from build123d import *

# Parameters (mm, degrees)
BOSS_EXTRUDE7_DEPTH = 3
SKETCH12_R          = 1.15
CUT_EXTRUDE3_DEPTH  = 75.228296491
SKETCH11_R          = 1.45
CUT_EXTRUDE4_DEPTH  = 75.228296491
SKETCH13_R          = 1.15
CUT_EXTRUDE5_DEPTH  = 75.228296491
FILLET1_R           = 4.7
FILLET2_R           = 3.8


with BuildPart() as part:
    # Sketch10 → Boss-Extrude7 (new body)
    with BuildSketch(Plane.XY):
        Polygon((22.4, 10.2), (62.6, 10.2), (62.6, -10.2), (72, -10.2), (72, 17.8), (8, 17.8), (8, 10.2), (-8, 10.2), (-8, 5), (8, 5), (8, -5), (-8, -5), (-8, -10.2), (22.4, -10.2), align=None)
    extrude(amount=-BOSS_EXTRUDE7_DEPTH)

    # Sketch12 → Cut-Extrude3 (cut, through all)
    with BuildSketch(Plane(origin=(0, 0, 0), x_dir=(-1, 0, 0), z_dir=(0, 0, -1))):
        with Locations((-57.5, 12.7)):
            Circle(SKETCH12_R)
        with Locations((-47.5, 12.7)):
            Circle(SKETCH12_R)
    extrude(amount=CUT_EXTRUDE3_DEPTH, mode=Mode.SUBTRACT)

    # Sketch11 → Cut-Extrude4 (cut, through all)
    with BuildSketch(Plane(origin=(0, 0, 0), x_dir=(-1, 0, 0), z_dir=(0, 0, -1))):
        with Locations((-67.3, -5)):
            Circle(SKETCH11_R)
        with Locations((-17.7, -5)):
            Circle(SKETCH11_R)
        with Locations((-17.7, 5)):
            Circle(SKETCH11_R)
        with Locations((-67.3, 5)):
            Circle(SKETCH11_R)
    extrude(amount=CUT_EXTRUDE4_DEPTH, mode=Mode.SUBTRACT)

    # Sketch13 → Cut-Extrude5 (cut, through all)
    with BuildSketch(Plane.XY):
        with Locations((5, 7.6)):
            Circle(SKETCH13_R)
        with Locations((5, -7.6)):
            Circle(SKETCH13_R)
    extrude(amount=-CUT_EXTRUDE5_DEPTH, mode=Mode.SUBTRACT)

    # Fillet1
    fillet1_edges = [part.edges().sort_by_distance(p)[0] for p in [
        (72, 17.8, -1.5),
        (72, -10.2, -1.5),
    ]]
    fillet(fillet1_edges, radius=FILLET1_R)

    # Fillet2
    fillet2_edges = [part.edges().sort_by_distance(p)[0] for p in [
        (22.4, -10.2, -1.5),
        (-8, -10.2, -1.5),
        (8, 17.8, -1.5),
        (8, 10.2, -1.5),
        (-8, 10.2, -1.5),
    ]]
    fillet(fillet2_edges, radius=FILLET2_R - 0.0001)  # a hair under: the kernel refuses the full size


solid = part.part
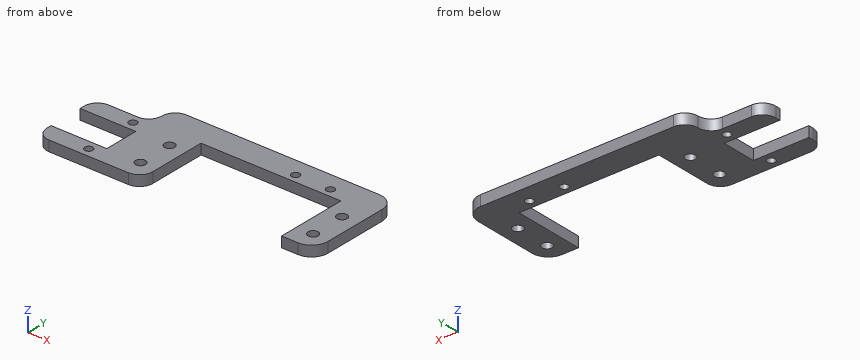
Geometry check sheet. Reference: the model listing, model coordinates, mm. Round coordinates to 2 decimals unless told otherwise and drop trailing zeros. Order: outer loops, then holes, each group sorted by start corner. A loop starts at its lowest first (then second) coordinate and runs counter-clockwise, first axis right, second up. Notation, with made-up numbers: M 76.25,65 L 101.25,65 A15 ccw 101.25,82 Z; hole C 47.25,44.5 d4. An arc over 180 degrees is marked long. Answer in a Markdown table with one row per item. Add a question column.
Item 1: Sectioned sample at D-D, the plane y = 7.6. Enter the section's corners in (x, z).
Item 2: Sectioned sample at C-C, the plane y = -2. Enter the section's corners in (x, z), plus the area to 3 significant figures.
Item 3: Sectioned sample at A-A, the plane x = 57.5. Enter the section's corners in (y, z), plus the area to 3 significant figures.
Item 4: Sectioned sample at B-B, the plane z = -1.5. State how many separate pieces and enclosed holes the cut face has, plus the area to 3 significant figures.
Item 5: Material ranges on L1, parallel to Y at x = 17.7, z = -1; L2, parallel to Y at x = 1, z = -2.1; L3, parallel to X at y = 12.7, z = -1.5, recorded low to high. Write a range as [from, to].
Item 6: Depth check by flat-ended pin: pin 1 Ø1.5 at (x, z) = (41.5, -1) entering from -Y; pin 2 Ø2.5 at (x, y) = (17.7, 5) entering from -Z; pin 3 Ø0.9 at (y, z) = (-3, -1.5) entering from -X; pin 4 Ø1 at (y, z) = (13, -1.5) entering from -X. Enter the tip coordinate at first touch or a pass-through.
Filled in:
| question | item | result |
|---|---|---|
| 1 | outline | M -7.81,-3 L 3.85,-3 L 3.85,0 L -7.81,0 Z; M 6.15,-3 L 22.4,-3 L 22.4,0 L 6.15,0 Z; M 62.6,-3 L 72,-3 L 72,0 L 62.6,0 Z |
| 2 | outline | M 8,-3 L 22.4,-3 L 22.4,0 L 8,0 Z; M 62.6,-3 L 72,-3 L 72,0 L 62.6,0 Z |
| 2 | area | 71.4 mm² |
| 3 | outline | M 10.2,-3 L 11.55,-3 L 11.55,0 L 10.2,0 Z; M 13.85,-3 L 17.8,-3 L 17.8,0 L 13.85,0 Z |
| 3 | area | 15.9 mm² |
| 4 | separate pieces | 1 |
| 4 | enclosed holes | 8 |
| 4 | area | 1,080 mm² |
| 5 | L1 | y = [-10.2, -6.45], [-3.55, 3.55], [6.45, 17.8] |
| 5 | L2 | y = [-10.2, -5], [5, 10.2] |
| 5 | L3 | x = [7.77, 46.35], [48.65, 56.35], [58.65, 72] |
| 6 | pin 1 | stops at y = 10.2 |
| 6 | pin 2 | passes through |
| 6 | pin 3 | stops at x = 8 |
| 6 | pin 4 | stops at x = 7.69 |
